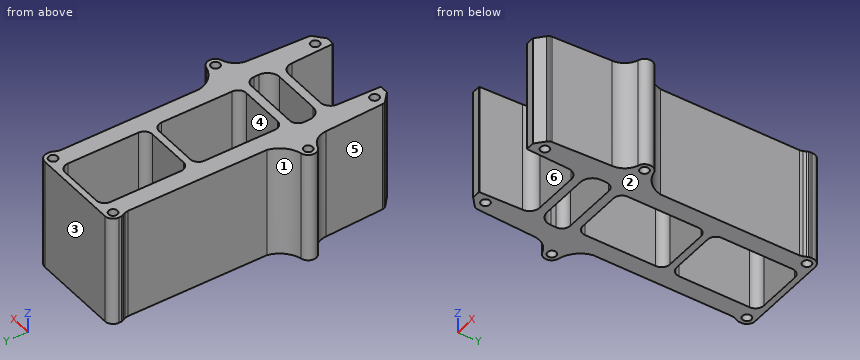
```python
from build123d import *

# Parameters (mm, degrees)
F0_R     = 2.3945844673
F1_DEPTH = 60
F3_SCALE = 0.6563


with BuildPart() as f1:
    # F0 (on Top) → F1 (new body)
    with BuildSketch(Plane.XY):
        with BuildLine():
            Line((-27.0389984867, 83.2772081509), (-26.4251961202, 81.9096698061))
            Line((-26.4251961202, 81.9096698061), (-26.0784868151, 80.2167370168))
            Line((-26.0784868151, 80.2167370168), (-26.0784868151, 5.1366092342))
            ThreePointArc((-26.0784868151, 5.1366092342), (-29.7252239834, -1.8462109586), (-36.4788286904, -5.9017372231))
            ThreePointArc((-36.4788286904, -5.9017372231), (-40.3150914077, -10.07792875), (-36.9143450669, -14.6158150015))
            ThreePointArc((-36.9143450669, -14.6158150015), (-32.1922887959, -18.1949867477), (-30.2764291391, -23.8019259832))
            Line((-30.2764291391, -23.8019259832), (-28.8915335984, -55.4398973488))
            Line((-28.8915335984, -55.4398973488), (-28.7443264889, -56.2413544219))
            Line((-28.7443264889, -56.2413544219), (-28.3286040912, -57.0579545856))
            Line((-28.3286040912, -57.0579545856), (-27.844521729, -57.4991165442))
            Line((-27.844521729, -57.4991165442), (-23.1986730857, -61.6394566898))
            Line((-23.1986730857, -61.6394566898), (-22.8441298419, -61.7180224508))
            Line((-22.8441298419, -61.7180224508), (-18.6802665162, -61.7180224508))
            Line((-18.6802665162, -61.7180224508), (-18.4410806307, -61.4369034612))
            Line((-18.4410806307, -61.4369034612), (-17.6754507656, -38.8146494524))
            ThreePointArc((-17.6754507656, -38.8146494524), (-16.0548504259, -34.9431431488), (-12.175320372, -33.3418458372))
            Line((-12.175320372, -33.3418458372), (0.0142386856, -33.3418458372))
            Line((0.0142386856, -33.3418458372), (0.0142386856, -28.883429572))
            Line((0.0142386856, -28.883429572), (-12.867449671, -28.883429572))
            ThreePointArc((-12.867449671, -28.883429572), (-17.4637841926, -26.979565476), (-19.3676482886, -22.3832309544))
            Line((-19.3676482886, -22.3832309544), (-19.3676482886, -19.4763654619))
            ThreePointArc((-19.3676482886, -19.4763654619), (-18.0495706302, -16.2942445028), (-14.867449671, -14.9761668444))
            Line((-14.867449671, -14.9761668444), (0.0142386856, -14.9761668444))
            Line((0.0142386856, -14.9761668444), (0.0142386856, -10.3005459473))
            Line((0.0142386856, -10.3005459473), (-11.9863399565, -10.3005459473))
            ThreePointArc((-11.9863399565, -10.3005459473), (-15.1684609157, -8.9824682889), (-16.4865385741, -5.8003473297))
            Line((-16.4865385741, -5.8003473297), (-16.4865385741, 32.2654335052))
            ThreePointArc((-16.4865385741, 32.2654335052), (-15.1684609157, 35.4475544644), (-11.9863399565, 36.7656321228))
            Line((-11.9863399565, 36.7656321228), (0.0142386856, 36.7656321228))
            Line((0.0142386856, 36.7656321228), (0.0142386856, 40.4444549151))
            Line((0.0142386856, 40.4444549151), (-11.9852216709, 40.4444549151))
            ThreePointArc((-11.9852216709, 40.4444549151), (-15.1673426301, 41.7625325735), (-16.4854202885, 44.9446535327))
            Line((-16.4854202885, 44.9446535327), (-16.4854202885, 83.0104343675))
            ThreePointArc((-16.4854202885, 83.0104343675), (-15.1673426301, 86.1925553267), (-11.9852216709, 87.5106329851))
            Line((-11.9852216709, 87.5106329851), (0.0142386856, 87.5106329851))
            Line((0.0142386856, 87.5106329851), (0.0142386856, 90.6373629034))
            Line((0.0142386856, 90.6373629034), (-23.213673197, 90.6373629034))
            ThreePointArc((-23.213673197, 90.6373629034), (-26.4197034776, 89.2897278228), (-27.6474967488, 86.0359186467))
            Line((-27.6474967488, 86.0359186467), (-27.6474967488, 84.8186316031))
            Line((-27.6474967488, 84.8186316031), (-27.4746276334, 84.2558386951))
            Line((-27.4746276334, 84.2558386951), (-27.0389984867, 83.2772081509))
        make_face()
        with Locations((-23.0123251677, -55.1256909966)):
            Circle(F0_R, mode=Mode.SUBTRACT)
        with Locations((-35.8826853335, -10.2994536757)):
            Circle(F0_R, mode=Mode.SUBTRACT)
        with Locations((-23.2493666078, 86.2348794977)):
            Circle(F0_R, mode=Mode.SUBTRACT)
    extrude(amount=F1_DEPTH)

    # F2: F1 across plane


with BuildPart() as f1_1:
    add(f1.part)
    add(f1.part.mirror(Plane.YZ))


with BuildPart() as f1_2:
    # F3: moved
    add(f1_1.part.scale(F3_SCALE).moved(Location((0.5205121011, -3.0246793772, 0))))


solid = f1_2.part
```
Model file for the job. Use its own axes, mm. Face numbers are marked on the shaded views. A direction names the side the tool comes from. Give positions to 0.01 mm unless a question says otherwise; leave off trailing zeros. Loops run counter-clockwise (first coordinate to the right, second up) from the corner with the lowest first, then second, coordinate; pieces in that order, holes last. Notation, with made-up numbers: (-20, 40) -> (12, 40) arc R20 ccw to (12, 62) -> close; hole circle Ø4 at (73.25, 87). An arc over 180 degrees is marked (long way). Write each question's results on one line, items separated by ' | '.
(1) Probe line 1 along Y through (x, z) = (7, 24); line 2 along Y through (x, z) = (10.5, 5); line 3 along X through (y, z) = (2.5, 10.5). List the from-to ranges inside material, lowest first.
Geometry results:
line 1: y = -24.91 to -21.98, -12.85 to -9.78, 21.1 to 23.52, 54.41 to 56.46 | line 2: y = -25.5 to -21.7, -12.86 to -8.9, 20.21 to 24.41, 53.52 to 56.46 | line 3: x = -16.59 to -10.3, 11.34 to 17.64
(2) Pull direction Y, two halves, no side cores. Call the marked faces 1, 2 and 3: released by +Y, released by -Y, zero draft, split by the parting line, or undercut.
Geometry results:
face 1: undercut | face 2: zero draft | face 3: released by +Y
(3) Tool access for the marked faces 4, 5 and 6: list every direction of +Z, -Z, +X, -X, +Y, -Y with a clear straight run to the whole face (end or side of a thin tool).
Geometry results:
face 4: +Z, -Z | face 5: +Z, -Z, -X, -Y | face 6: +Z, -Z, -Y
(4) Flat gauge pins, fed straight in: pin 1 Ø10 at (y, z) = (36, 24) entering from +X; pin 2 Ø0.9 at (y, z) = (53, 24.5) entering from +X; pin 3 Ø20 at (y, z) = (5, 28.5) entering from -X. Where does each tip first touch, or does it go through?
Geometry results:
pin 1: stops at x = 17.64 | pin 2: stops at x = 18.67 | pin 3: stops at x = -19.8
(5) Cut at A-A on x = 2.5. List the corners of the cut face in (y, z), and give its area (3 significant figures).
Geometry results:
outline: (-24.91, 0) -> (-21.98, 0) -> (-21.98, 39.38) -> (-24.91, 39.38) -> close; (-12.85, 0) -> (-9.78, 0) -> (-9.78, 39.38) -> (-12.85, 39.38) -> close; (21.1, 0) -> (23.52, 0) -> (23.52, 39.38) -> (21.1, 39.38) -> close; (54.41, 0) -> (56.46, 0) -> (56.46, 39.38) -> (54.41, 39.38) -> close | area: 412 mm²
(6) Cut at C-C on y = -32.5. List the corners of the cut face in (x, z), and give its area (3 significant figures).
Geometry results:
outline: (-18.74, 0) -> (-11.22, 0) -> (-11.22, 39.38) -> (-18.74, 39.38) -> close; (12.26, 0) -> (19.78, 0) -> (19.78, 39.38) -> (12.26, 39.38) -> close | area: 593 mm²
(7) Cut at D-D on z = 15. Give the number of separate pieces and of enclosed holes in the cut face, and give its area (3 significant figures).
Geometry results:
separate pieces: 1 | enclosed holes: 9 | area: 1,680 mm²
(8) Cut at B-B on y = 48. List the corners of the cut face in (x, z), and give its area (3 significant figures).
Geometry results:
outline: (-16.59, 0) -> (-10.3, 0) -> (-10.3, 39.38) -> (-16.59, 39.38) -> close; (11.34, 0) -> (17.64, 0) -> (17.64, 39.38) -> (11.34, 39.38) -> close | area: 496 mm²
